Job drawing, mm, ordinate dimensions from the low corner. One solid piece. A direction names the side the tool comes from. Round coordinates to 2 decimals unless told otherwise and drop trailing zeros. Order: outer loops, then holes, each group sorted by start corner. A loop starts at its lowest first (then second) coordinate and runs counter-clockwise, first axis right, second up. Notation, with made-up numbers: (39.5, 47.25) -> (53.5, 47.25) arc R35 cw to (53.5, 85.25) -> close; hole circle Ø3 at (-32, 56). An arc over 180 degrees is marked (long way). Return JSON: item names as keys, results as strings. Group by question number.
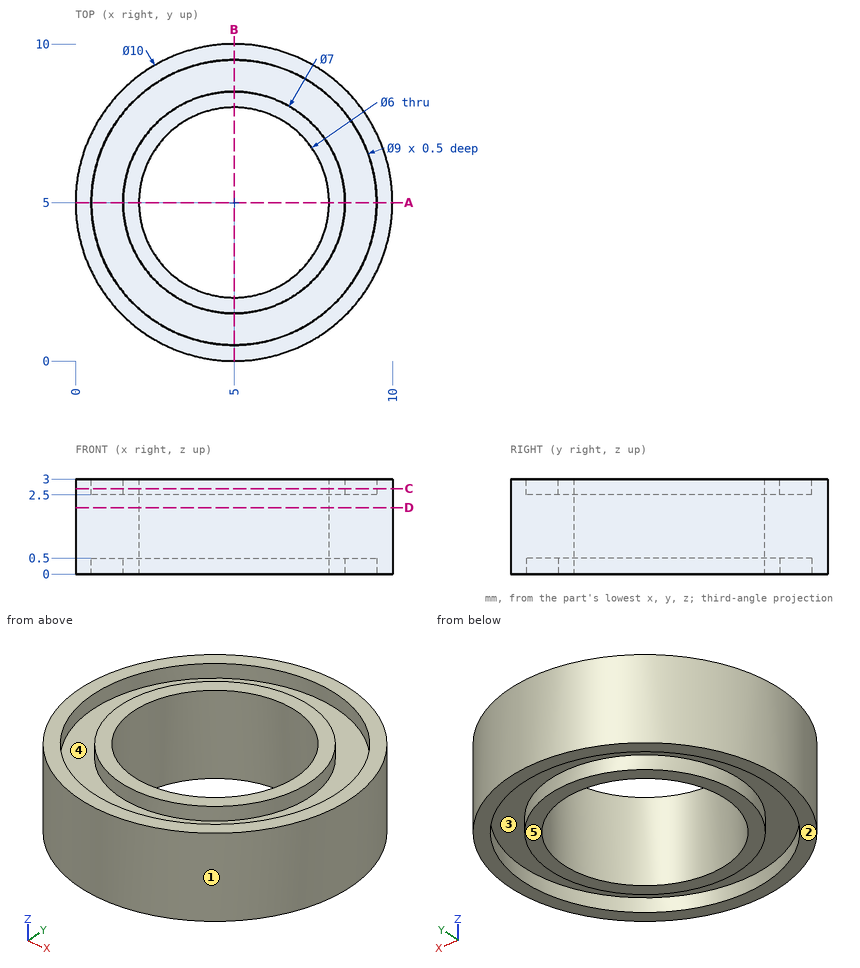
(1) Saw through at D-D, the plane z = 2.1. List the corners of the cut face in (x, y), and give its area (3 significant figures).
(2) Saw through at A-A, the plane y = 5. List the corners of the cut face in (x, z), and give its area (3 significant figures).
(3) Probe L1, parallel to Y at x = 5, z = 2.75; L2, parallel to Y at x = 5, z = 2.1; L3, parallel to Y at x = 3, z = 2.55. List the from-to ranges inside material, lowest first. Write a range as [from, to].
(4) Tool access for the marked faces 4 and 5: list every direction of +Z, -Z, +X, -X, +Y, -Y with a clear straight run to the whole face (end or side of a thin tool).
(5) Pin check, flat tips, straight feed: P1, Ø1, axis at y = 6, z = 1, coming from the -X side; P2, Ø1.5, axis at x = 2, z = 1.5, coming from the +Y side; P3, Ø4.5, axis at x = 4.5, y = 3, coming from the +Z side; P4, Ø1, axis at y = 2.5, z = 2, coming from the -X side. Stop position of each tip, or through.
(6) Mould opens along Y. For the marked faces 1, 2 and 3 say: pulls with the +Y half, pulls with the -Y half, needs draft (parallel to the pull), parting line crosses it, or undercut.
(7) Saw through at C-C, the plane z = 2.7. List the corners of the cut face in (x, y).
Results are:
{
 "1": {"outline": "circle Ø10 at (5, 5); hole circle Ø6 at (5, 5)", "area": "50.3 mm^2"},
 "2": {"outline": "(0, 0) -> (0.5, 0) -> (0.5, 0.5) -> (1.5, 0.5) -> (1.5, 0) -> (2, 0) -> (2, 3) -> (1.5, 3) -> (1.5, 2.5) -> (0.5, 2.5) -> (0.5, 3) -> (0, 3) -> close; (8, 0) -> (8.5, 0) -> (8.5, 0.5) -> (9.5, 0.5) -> (9.5, 0) -> (10, 0) -> (10, 3) -> (9.5, 3) -> (9.5, 2.5) -> (8.5, 2.5) -> (8.5, 3) -> (8, 3) -> close", "area": "10.0 mm^2"},
 "3": {"L1": "y = [0, 0.5], [1.5, 2], [8, 8.5], [9.5, 10]", "L2": "y = [0, 2], [8, 10]", "L3": "y = [0.42, 0.97], [2.13, 2.76], [7.24, 7.87], [9.03, 9.58]"},
 "4": {"face 4": "+Z", "face 5": "-Z, +X, -X, +Y, -Y"},
 "5": {"P1": "stops at x = 0.03", "P2": "stops at y = 9.47", "P3": "stops at z = 3", "P4": "stops at x = 0.42"},
 "6": {"face 1": "parting line crosses it", "face 2": "needs draft", "face 3": "undercut"},
 "7": {"outline": "circle Ø10 at (5, 5); circle Ø7 at (5, 5); hole circle Ø9 at (5, 5); hole circle Ø6 at (5, 5)"}
}
